from build123d import *

# Parameters (mm, degrees)
BOSS_EXTRUDE1_DEPTH = 26.65
BOSS_EXTRUDE2_DEPTH = 1.25
BOSS_EXTRUDE3_DEPTH = 1.25
SKETCH4_R           = 3
CUT_EXTRUDE1_DEPTH  = 1.25
SKETCH5_R           = 3
CUT_EXTRUDE2_DEPTH  = 1.25
SKETCH6_W           = 35.469315919
SKETCH6_H           = 20.901561166
CUT_EXTRUDE3_DEPTH  = 1.25
CUT_EXTRUDE4_DEPTH  = 1.25
CUT_EXTRUDE5_DEPTH  = 41.25


with BuildPart() as part:
    # Sketch1 → Boss-Extrude1 (new body)
    with BuildSketch(Plane(origin=(0, 0, 0), x_dir=(1, 0, 0), z_dir=(0, 1, 0))):
        Polygon((65.740483752, 35.768961664), (-16.155551111, 5.899521732), (-49.97807415, -42.47004645), (-51.002473848, -41.753732791), (-16.954107408, 6.938813892), (65.312177163, 36.943292736), align=None)
    extrude(amount=BOSS_EXTRUDE1_DEPTH)

    # Sketch2 → Boss-Extrude2 (add)
    with BuildSketch(Plane(origin=(0, 26.65, 0), x_dir=(1, 0, 0), z_dir=(0, 1, 0))):
        Polygon((-51.002473848, -41.753732791), (-49.97807415, -42.47004645), (-7.877469848, -6.485888625), (65.740483752, 35.768961664), (65.312177163, 36.943292736), (-16.954107408, 6.938813892), align=None)
    extrude(amount=BOSS_EXTRUDE2_DEPTH)

    # Sketch3 → Boss-Extrude3 (add)
    with BuildSketch(Plane.XZ):
        Polygon((65.312177163, -36.943292736), (65.740483752, -35.768961664), (-7.877469848, 6.485888625), (-49.97807415, 42.47004645), (-51.002473848, 41.753732791), (-16.954107408, -6.938813892), align=None)
    extrude(amount=BOSS_EXTRUDE3_DEPTH)

    # Sketch4 → Cut-Extrude1 (cut)
    with BuildSketch(Plane(origin=(-4.224136578, 0, -11.581738298), x_dir=(-0.9394648571224508, 0, 0.34264527171973835), z_dir=(-0.34264527171973835, 0, -0.9394648571224508))):
        with Locations((-68.516939764, 21.15)):
            Circle(SKETCH4_R)
        with Locations((-37.516939764, 21.15)):
            Circle(SKETCH4_R)
        with Locations((-37.516939764, 5.5)):
            Circle(SKETCH4_R)
        with Locations((-68.516939764, 5.5)):
            Circle(SKETCH4_R)
    extrude(amount=-CUT_EXTRUDE1_DEPTH, mode=Mode.SUBTRACT)

    # Sketch5 → Cut-Extrude2 (cut)
    with BuildSketch(Plane(origin=(-14.645244024, 0, -10.240717915), x_dir=(-0.5730509275214783, 0, 0.819519758435862), z_dir=(-0.819519758435862, 0, -0.5730509275214783))):
        with Locations((57.095023955, 21.15)):
            Circle(SKETCH5_R)
        with Locations((57.095023955, 5.5)):
            Circle(SKETCH5_R)
    extrude(amount=-CUT_EXTRUDE2_DEPTH, mode=Mode.SUBTRACT)

    # Sketch6 → Cut-Extrude3 (cut)
    with BuildSketch(Plane(origin=(-14.645244024, 0, -10.240717915), x_dir=(-0.5730509275214783, 0, 0.819519758435862), z_dir=(-0.819519758435862, 0, -0.5730509275214783))):
        with Locations((30.344239524, 13.325)):
            Rectangle(SKETCH6_W, SKETCH6_H)
    extrude(amount=-CUT_EXTRUDE3_DEPTH, mode=Mode.SUBTRACT)

    # Sketch7 → Cut-Extrude4 (cut)
    with BuildSketch(Plane(origin=(-4.224136578, 0, -11.581738298), x_dir=(-0.9394648571224508, 0, 0.34264527171973835), z_dir=(-0.34264527171973835, 0, -0.9394648571224508))):
        Polygon((-13.799604913, 23.775780583), (-7.799604913, 23.775780583), (-7.799604913, 2.874219417), (-13.799604913, 2.874219417), (-30.928783923, 2.874219417), (-30.928783923, 23.775780583), align=None)
    extrude(amount=-CUT_EXTRUDE4_DEPTH, mode=Mode.SUBTRACT)

    # Sketch8 → Cut-Extrude5 (cut)
    with BuildSketch(Plane.XZ.offset(1.25)):
        Polygon((65.740483752, -35.768961664), (-9.082823105, 4.70312394), (-49.97807415, 42.47004645), (-7.877469848, 6.485888625), align=None)
    extrude(amount=-CUT_EXTRUDE5_DEPTH, mode=Mode.SUBTRACT)


solid = part.part
Source: CAD feature listing. Evaluate the final solid. Frame: model axes, mm. A direction names the side the tool comes from. Coordinates: 2 decimals unless noted, no trailing zeros. Loops run counter-clockwise (first coordinate to the right, second up) from the corner with the lowest first, then second, coordinate; pieces in that order, holes last. Notation, with made-up numbers: (63.25, 89.5) -> (110.25, 89.5) arc R19 ccw to (110.25, 117.5) -> close; hole circle Ø6 at (81, -31). An arc over 180 degrees is marked (long way). Answer in a Markdown table with one row per item. Add a question column.
Q1. Pull-direction query (X, two-part tool) for faces 3 (the face through (-38, 26.48, 23.16)), 4 (the face through (29.9, 18.5, -23.4)), 5 (the face through (-1, 26.65, -3)); classes: pulls with the +X half, pulls with the -X half, needs draft (parallel to the pull), parting line crosses it, or undercut.
Q2. Section C-C on z = -16. Return the cut outline in (x, y).
Q3. Section D-D on x = 46. Return the cut outline in (y, z).
Q4. Ray query, line 1 along Y through (x, z) = (2, -11); line 2 along Y through (x, z) = (-24, 4.5); line 3 along Z through (x, y) = (54.5, 14). Return the intervals inside material, ascending.
Q5. Reachability of faces 1 (the face through (-1, 0, -2)), 2 (the face through (-2, 27.9, -3)) from +Z, -Z, +X, -X, +Y, -Y: full face, straight path, thin tool, end or side. Return the list, or none.
Q6. Section B-B on x = -28. Return the cut outline in (y, z).
Q7. Section A-A on y = 10.25. Return the cut outline in (x, z) (1 decimal), and give its area (3 significant figures).
Q8. Contact query for flat-ended pins moving along their axis: pin 1 Ø4 at (x, y) = (25, 8) entering from -Z; pin 2 Ø6 at (y, z) = (7.5, -17) entering from +X; pin 3 Ø8 at (x, y) = (-9.5, 3.5) entering from -Z. Output: stop coordinate, or through.
Computed values:
| question | item | result |
|---|---|---|
| 1 | face 3 | pulls with the -X half |
| 1 | face 4 | undercut |
| 1 | face 5 | needs draft |
| 2 | outline | (7.89, -1.25) -> (29.19, -1.25) -> (29.19, 0) -> (11.54, 0) -> (11.54, 2.87) -> (7.89, 2.87) -> close; (7.89, 23.78) -> (11.54, 23.78) -> (11.54, 26.65) -> (29.19, 26.65) -> (29.19, 27.9) -> (7.89, 27.9) -> close |
| 3 | outline | (-1.25, -29.9) -> (27.9, -29.9) -> (27.9, -25.09) -> (26.65, -25.09) -> (26.65, -28.57) -> (0, -28.57) -> (0, -25.09) -> (-1.25, -25.09) -> close |
| 4 | line 1 | y = -1.25 to 0, 26.65 to 27.9 |
| 4 | line 2 | y = -1.25 to 2.87, 23.78 to 27.9 |
| 4 | line 3 | z = -33 to -31.67 |
| 5 | face 1 | +Z, +X |
| 5 | face 2 | +Z, -Z, +X, -X, +Y |
| 6 | outline | (-1.25, 8.86) -> (2.87, 8.86) -> (2.87, 11.04) -> (0, 11.04) -> (0, 22.17) -> (-1.25, 22.17) -> close; (23.78, 8.86) -> (27.9, 8.86) -> (27.9, 22.17) -> (26.65, 22.17) -> (26.65, 11.04) -> (23.78, 11.04) -> close |
| 7 | outline | (-51, 41.8) -> (-42.2, 29.2) -> (-41.2, 29.9) -> (-50, 42.5) -> close; (-21.9, 0.1) -> (-17, -6.9) -> (3.1, -14.3) -> (3.5, -13.1) -> (-16.2, -5.9) -> (-20.8, 0.8) -> close; (24.8, -22.2) -> (65.3, -36.9) -> (65.7, -35.8) -> (25.3, -21) -> close |
| 7 | area | 110 mm^2 |
| 8 | pin 1 | stops at z = -22.97 |
| 8 | pin 2 | stops at x = 3.2 |
| 8 | pin 3 | stops at z = -11.12 |
